Geometry check sheet. Reference: drawing and pictorial views, mm from the part's lowest x, y, z. A direction names the side the tool comes from. Give positions to 0.01 mm unless a question says otherwise; leave off trailing zeros. Order: outer loops, then holes, each group sorted by start corner. A loop starts at its lowest first (then second) coordinate and runs counter-clockwise, first axis right, second up.
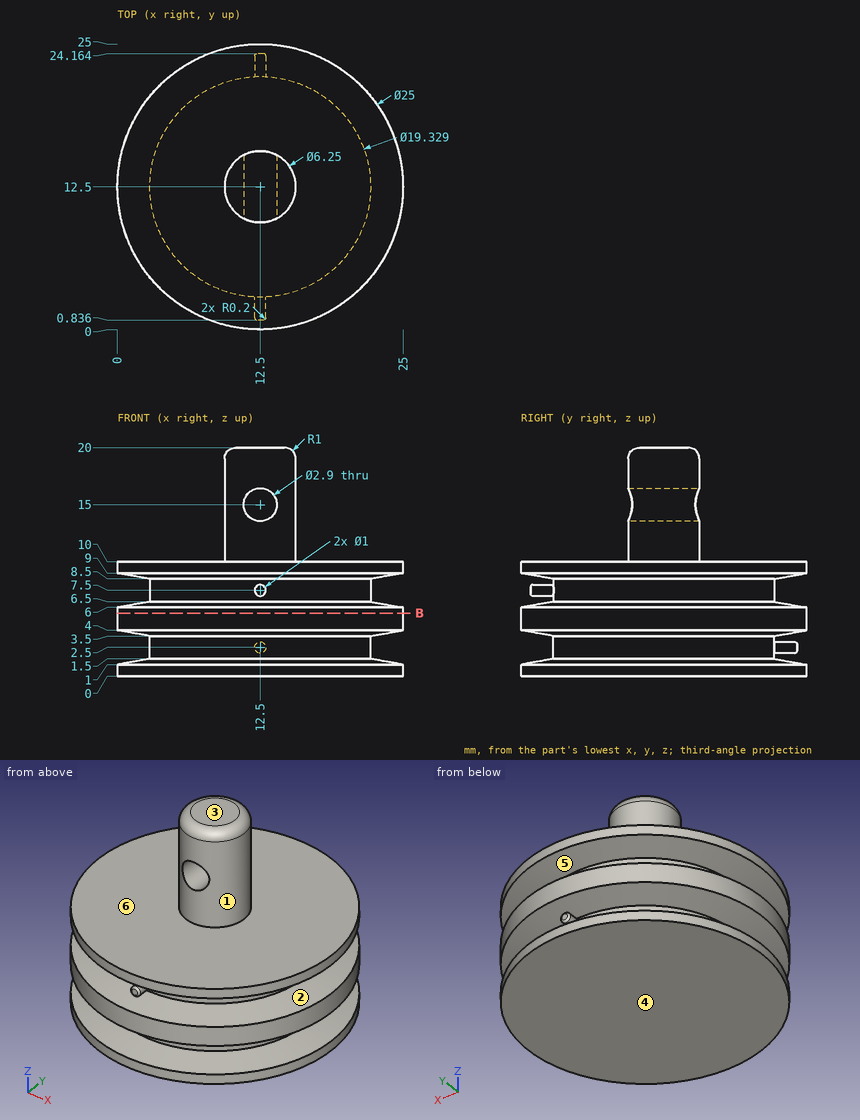
(1) Material ranges on L1, parallel to Z at x = 12.5, y = 11; L2, parallel to Z at x = 2, y = 15.75; L3, parallel to Z at x = 8.5, y = 3.5, recorded low to high.
Response values:
L1: z = 0 to 13.55, 16.45 to 20
L2: z = 0 to 1.27, 3.73 to 6.27, 8.73 to 10
L3: z = 0 to 1.47, 3.53 to 6.47, 8.53 to 10
(2) Cross-section at B-B on z = 5.5. Enter the section's corners in (x, y).
Response values:
outline: circle Ø25 at (12.5, 12.5)
(3) Set-up check for the marked faces 1, 2 and 3: record each of +Z, -Z, +X, -X, +Y, -Y from which the full face is reachable in a straight line by a thin tool's end or side.
Response values:
face 1: +Z
face 2: none
face 3: +Z, +X, -X, +Y, -Y
(4) Gauge pin test, flat ends, axial feed: pin 1 Ø3 at (x, y) = (22, 2.5) entering from +Z; pin 2 Ø2 at (x, z) = (7.5, 10.5) entering from +Y; pin 3 Ø2 at (y, z) = (13.5, 3.5) entering from +X; pin 4 Ø1.7 at (x, z) = (12.5, 15) entering from -Y. Record the tip position at first contact, or that the pin passes through.
Response values:
pin 1: stops at z = 10
pin 2: stops at y = 24.3
pin 3: stops at x = 25
pin 4: passes through
(5) Release check for a two-part mould opening along Z. For the marked faces 4, 5 and 6 record: released by +Z, released by -Z, zero draft, split by the parting line, or undercut.
Response values:
face 4: released by -Z
face 5: undercut
face 6: released by +Z
